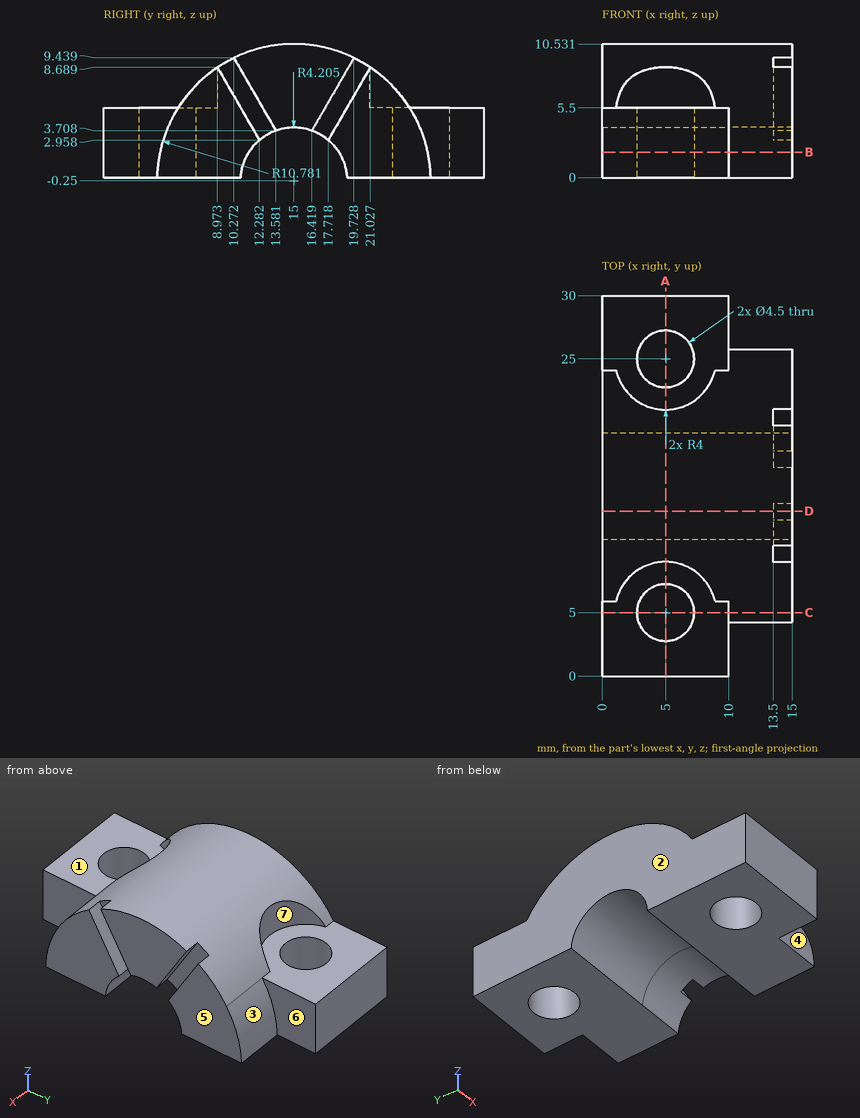
Could you check a few things on this drawing? It's one solid part, dimensions in mm from its lowest x, y, z. A direction names the side the tool comes from. Coordinates: 2 decimals unless noted, no trailing zeros. Loops run counter-clockwise (first coordinate to the right, second up) from the corner with the lowest first, then second, coordinate; pieces in that order, holes last. Notation, with made-up numbers: (-7, 89.25) - (43, 89.25) arc R19 cw to (43, 114.25) - close; hole circle Ø9 at (84, -35.5). An arc over 180 degrees is marked (long way). Return JSON: item names as keys, results as strings. Group by question number.
Item 1: If we section it at C-C on y = 5: Write out the boundary of the cut face in (x, z).
Item 2: If we section it at B-B on z = 2: Write out the boundary of the cut face in (x, y).
Item 3: On a 3-axis mill with a long thin cutter (end or side, diameter ignored), from which of +Z, -Z, +X, -X, +Y, -Y can I reach the whole of each face in a straight line? I mean the marked faces 4, 5, 6 and 7. Say none if no direction works.
Item 4: I need wall thicknesses on line 1 (X direction, y = 25, z = 3.55); line 2 (Y direction, x = 5, z = 1.95); line 3 (Y direction, x = 7, z = 5). Which ranges of each line are inside material? Lowest first, please. Write a range as from..to.
Item 5: Will these pins go through, and if not, where does the flat tip stop? P1, Ø3, axis at y = 27.5, z = 3.5, coming from the +X side; P2, Ø1.5, axis at y = 12.5, z = 1.5, coming from the -X side; P3, Ø2.5, axis at x = 3, y = 25, coming from the +Z side; P4, Ø4, axis at x = 1.5, y = 19, coming from the +Z side.
Item 6: If we section it at D-D on y = 13: Write out the boundary of the cut face in (x, z), and give its area (3 significant figures).
Item 7: If we section it at A-A on x = 5: State how many separate pieces and enclosed holes the cut face has, and give its area (3 significant figures).
Item 8: We'd pull the mould along X, two halves only. Please class the marked faces 1, 2 and 3: +X half, -X half, draft (parallel to the pull), parting line (faces both ways), or undercut.
Calculated:
{
 "1": {"outline": "(0, 0) - (2.75, 0) - (2.75, 5.5) - (0, 5.5) - close; (7.25, 0) - (15, 0) - (15, 3.78) - (10, 3.78) - (10, 5.5) - (7.25, 5.5) - close"},
 "2": {"outline": "(0, 0) - (10, 0) - (10, 4.46) - (15, 4.46) - (15, 11.45) - (0, 11.45) - close; (0, 18.55) - (15, 18.55) - (15, 25.54) - (10, 25.54) - (10, 30) - (0, 30) - close; hole circle Ø4.5 at (5, 5); hole circle Ø4.5 at (5, 25)"},
 "3": {"face 4": "+Z, +X, -Y", "face 5": "+Z, -Z, +X, +Y, -Y", "face 6": "+Z, +X, +Y", "face 7": "+Z, +Y"},
 "4": {"line 1": "x = 0..2.75, 7.25..15", "line 2": "y = 0..2.75, 7.25..11.42, 18.58..22.75, 27.25..30", "line 3": "y = 0..3.97, 6.03..23.97, 26.03..30"},
 "5": {"P1": "stops at x = 10", "P2": "passes through", "P3": "stops at z = 5.5", "P4": "stops at z = 10.34"},
 "6": {"outline": "(0, 3.45) - (13.5, 3.45) - (13.5, 4.71) - (15, 4.71) - (15, 10.34) - (0, 10.34) - close", "area": "102 mm^2"},
 "7": {"separate pieces": "3", "enclosed holes": "0", "area": "143 mm^2"},
 "8": {"face 1": "undercut", "face 2": "-X half", "face 3": "draft"}
}
